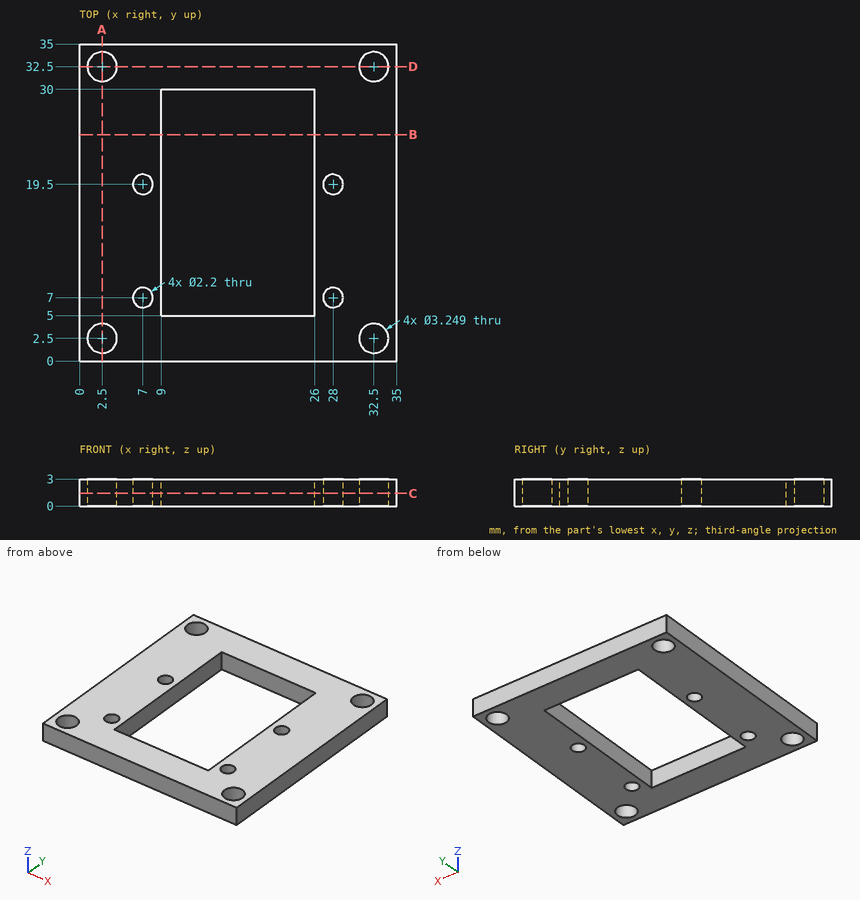
Print and shaded views of the part. All mm, measured from the part's lowest x, y and z. Round coordinates to 2 decimals unless told otherwise and drop trailing zeros. Loops run counter-clockwise (first coordinate to the right, second up) from the corner with the lowest first, then second, coordinate; pieces in that order, holes last. Notation, with made-up numbers: (-28.75, 3) -> (-6.75, 3) arc R13 ccw to (-6.75, 9) -> close; hole circle Ø1 at (24, 0). An arc over 180 degrees is marked (long way). Use CSV: the item, a comma, the result in double quotes. Start each with the question number.
1) Cut at A-A, the plane x = 2.5. Write the cut outline in (y, z) (1 decimal).
2) Cut at C-C, the plane z = 1.4. Give the number of separate pieces and of enclosed holes in the cut face.
3) Cut at B-B, the plane y = 25. Write the cut outline in (x, z), plus the area to 3 significant figures.
4) Drop flat-ended pins along their axis: P1, Ø2, axis at x = 7, y = 7, coming from the +Z side; P2, Ø2, axis at x = 8.5, y = 8, coming from the -Z side. Give the stop position or say it passes through.
5) Wall check: L1, parallel to Y at x = 2.5, z = 1.5 (1 decimal); L2, parallel to X at y = 21, z = 1.45; L3, parallel to Y at x = 33.5, z = 2.1. Give the ranges that are in metal, low to high. Write a range as [from, to].
Determined:
1,outline,"(0, 0) -> (0.9, 0) -> (0.9, 3) -> (0, 3) -> close; (4.1, 0) -> (30.9, 0) -> (30.9, 3) -> (4.1, 3) -> close; (34.1, 0) -> (35, 0) -> (35, 3) -> (34.1, 3) -> close"
2,separate pieces,"1"
2,enclosed holes,"9"
3,outline,"(0, 0) -> (9, 0) -> (9, 3) -> (0, 3) -> close; (26, 0) -> (35, 0) -> (35, 3) -> (26, 3) -> close"
3,area,"54.0 mm2"
4,P1,"passes through"
4,P2,"stops at z = 0"
5,L1,"y = [0, 0.9], [4.1, 30.9], [34.1, 35]"
5,L2,"x = [0, 9], [26, 35]"
5,L3,"y = [0, 1.22], [3.78, 31.22], [33.78, 35]"
